Can you work these out from the drawing? Everything is in mm from the part's minimum corner. Give positions to 0.01 mm unless a question says otherwise; leave off trailing zeros. Order: outer loops, then holes, each group sorted by start corner. A loop starts at its lowest first (then second) coordinate and runs counter-clockwise, first axis right, second up. Notation, with made-up numbers: (-7, 72.25) - (33, 72.25) arc R26 ccw to (33, 93.25) - close; hole circle Ø1 at (77, 12). An arc over 180 degrees is marked (long way). Answer as a JSON object with one key per item and string values.
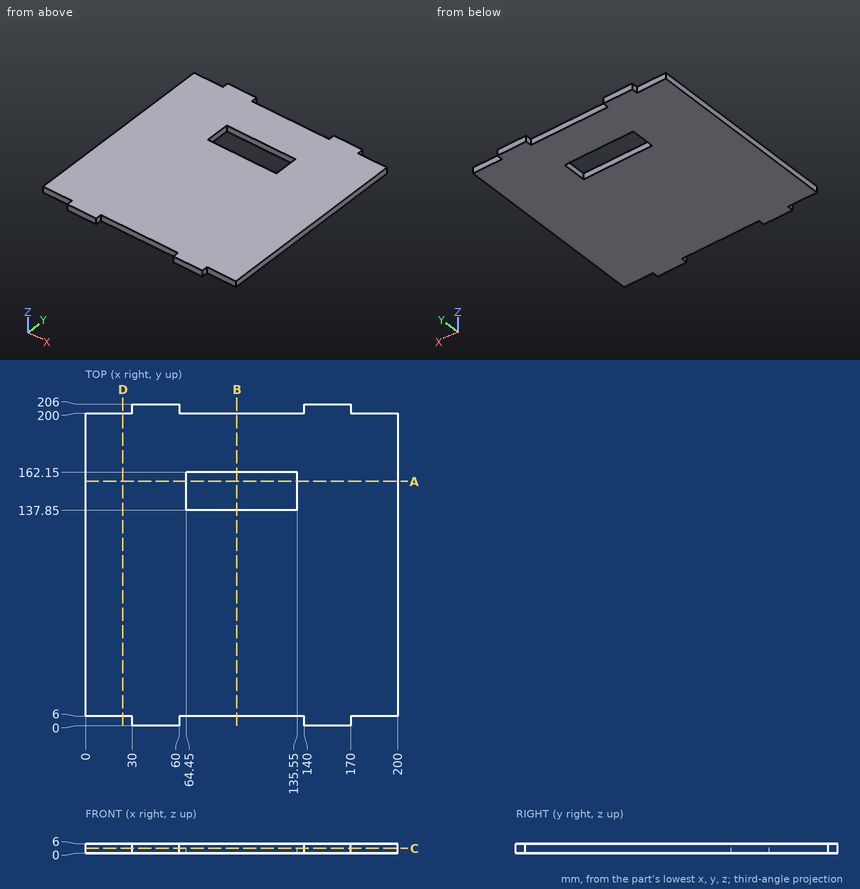
Q1. I need wall thicknesses on L1, parallel to Y at x = 65, z = 1.1; L2, parallel to X at y = 156.5, z = 2.2; L3, parallel to Y at x = 14, z = 0.8. Which ranges of each line are inside material? Lowest first, please.
Recorded:
{"L1": "y = 6 to 137.85, 162.15 to 200", "L2": "x = 0 to 64.45, 135.55 to 200", "L3": "y = 6 to 200"}
Q2. If we section it at D-D, the plane x = 24: Please give me the cut outline in (y, z).
Recorded:
{"outline": "(6, 0) - (200, 0) - (200, 6) - (6, 6) - close"}
Q3. If we section it at B-B, the plane x = 97: Please give me the cut outline in (y, z), then the cut area to 3 significant figures.
Recorded:
{"outline": "(6, 0) - (137.85, 0) - (137.85, 6) - (6, 6) - close; (162.15, 0) - (200, 0) - (200, 6) - (162.15, 6) - close", "area": "1,020 mm^2"}
Q4. If we section it at C-C, the plane z = 3.05: Please give me the cut outline in (x, y).
Recorded:
{"outline": "(0, 6) - (30, 6) - (30, 0) - (60, 0) - (60, 6) - (140, 6) - (140, 0) - (170, 0) - (170, 6) - (200, 6) - (200, 200) - (170, 200) - (170, 206) - (140, 206) - (140, 200) - (60, 200) - (60, 206) - (30, 206) - (30, 200) - (0, 200) - close; hole (64.45, 137.85) - (135.55, 137.85) - (135.55, 162.15) - (64.45, 162.15) - close"}
Q5. If we section it at A-A, the plane y = 156.5: Please give me the cut outline in (x, z).
Recorded:
{"outline": "(0, 0) - (64.45, 0) - (64.45, 6) - (0, 6) - close; (135.55, 0) - (200, 0) - (200, 6) - (135.55, 6) - close"}
Q6. I'm going to push flat-ended pins straight in: pin 1 Ø3 at (x, z) = (19.5, 3) entering from +Y; pin 2 Ø1.8 at (x, z) = (92, 2.5) entering from -Y; pin 3 Ø3 at (y, z) = (202.5, 4) entering from -X. Where does each tip first touch, or does it pass through?
Recorded:
{"pin 1": "stops at y = 200", "pin 2": "stops at y = 6", "pin 3": "stops at x = 30"}
